Geometry: final body of the model. Coordinates: model frame, mm. Round coordinates to 2 decimals unless told otherwise and drop trailing zeros. Loops run counter-clockwise (first coordinate to the right, second up) from the corner with the lowest first, then second, coordinate; pieces in that order, holes last. Notation, with made-up numbers: (-37.5, 51) -> (4.5, 51) arc R10 cw to (4.5, 58) -> close; hole circle Ø9 at (-31, -1). An arc over 180 degrees is marked (long way). Answer in a Markdown table with one row per item.
```python
from build123d import *

# Parameters (mm, degrees)
F1_DEPTH = 3.048


# Not quite as in the source:
# - ends of sketch curves that miss each other by under 0.0002 mm in the source are joined


with BuildPart() as f1:
    # F0 (on Top) → F1 (new body)
    with BuildSketch(Plane.XY):
        with BuildLine():
            Line((-234.6769754, 225.5266), (-280.958544, 225.5266))
            Line((-280.958544, 225.5266), (-280.958544, 149.1234))
            Line((-280.958544, 149.1234), (-235.1557146, 149.1234))
            Line((-235.1557146, 149.1234), (-119.0483268, 33.9200236))
            Line((-119.0483268, 33.9200236), (-119.0483268, -37.9720094))
            Line((-119.0483268, -37.9720094), (-166.0391904, -126.9183898))
            Line((-166.0391904, -126.9183898), (-235.6947534, -161.8234))
            Line((-235.6947534, -161.8234), (-280.958544, -161.8234))
            Line((-280.958544, -161.8234), (-280.958544, -225.5266))
            Line((-280.958544, -225.5266), (123.1089232, -225.5266))
            Line((123.1089232, -225.5266), (124.704856, -225.5266))
            Line((124.704856, -225.5266), (266.0774968, -225.5266))
            add(Edge.make_bspline(
                [(280.9585266998, -167.802566879), (240.6588540152, -189.7065906201), (266.0774968, -225.5266)],
                knots=[2.111008, 2.111008, 2.111008, 3.713127, 3.713127, 3.713127], degree=2, weights=[1, 0.6959462797, 1]))
            Line((280.9585266998, -167.802566879), (280.9585186, -167.27043))
            Line((280.9585186, -167.27043), (228.939217, -126.7947426))
            Line((228.939217, -126.7947426), (124.704856, 18.5980324))
            Line((124.704856, 18.5980324), (124.0087182, 19.2098422))
            Line((124.0087182, 19.2098422), (123.1089232, 20.0705212))
            Line((123.1089232, 20.0705212), (120.416701, 24.2140232))
            Line((120.416701, 24.2140232), (-40.9613862, 114.4633728))
            Line((-40.9613862, 114.4633728), (-234.6769754, 225.5266))
        make_face()
    extrude(amount=F1_DEPTH)


solid = f1.part
```
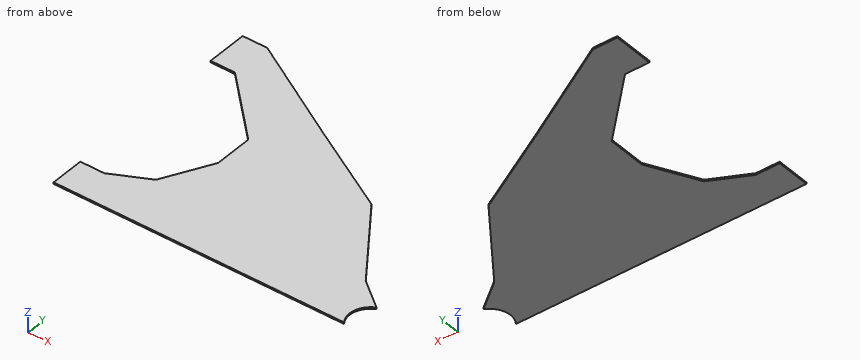
Item 1: Ray query, L1, parallel to Y at x = -19, z = 1.1; L2, parallel to X at y = -151.5, z = 0.85; L3, parallel to X at y = -97.5, z = 0.2. Return the intervals inside material, ascending.
Ans:
| item | result |
|---|---|
| L1 | -225.53 to 102.18 |
| L2 | -215.09 to 260.69 |
| L3 | -150.5 to 207.94 |
Item 2: Section query C-C, the plane x = -10.5. Output: boundary loops of the cut face in (y, z).
Ans:
| item | result |
|---|---|
| outline | (-225.53, 0) -> (97.43, 0) -> (97.43, 3.05) -> (-225.53, 3.05) -> close |
Item 3: Section query A-A, the plane x = -172. Output: boundary loops of the cut face in (y, z), and give its area (3 significant figures).
Ans:
| item | result |
|---|---|
| outline | (-225.53, 0) -> (-129.91, 0) -> (-129.91, 3.05) -> (-225.53, 3.05) -> close; (86.46, 0) -> (189.59, 0) -> (189.59, 3.05) -> (86.46, 3.05) -> close |
| area | 606 mm2 |
Item 4: Section query B-B, the plane y = -143. Output: boundary loops of the cut face in (x, z), and give its area (3 significant figures).
Ans:
| item | result |
|---|---|
| outline | (-198.13, 0) -> (249.77, 0) -> (249.77, 3.05) -> (-198.13, 3.05) -> close |
| area | 1,370 mm2 |
Item 5: First-contact query: P1, Ø1.5, axis at y = -12.5, z = 2.5, coming from the -X side. Flat tip, straight axial feed; report the tip coordinate or a pass-through.
Ans:
| item | result |
|---|---|
| P1 | x = -119.05 |
